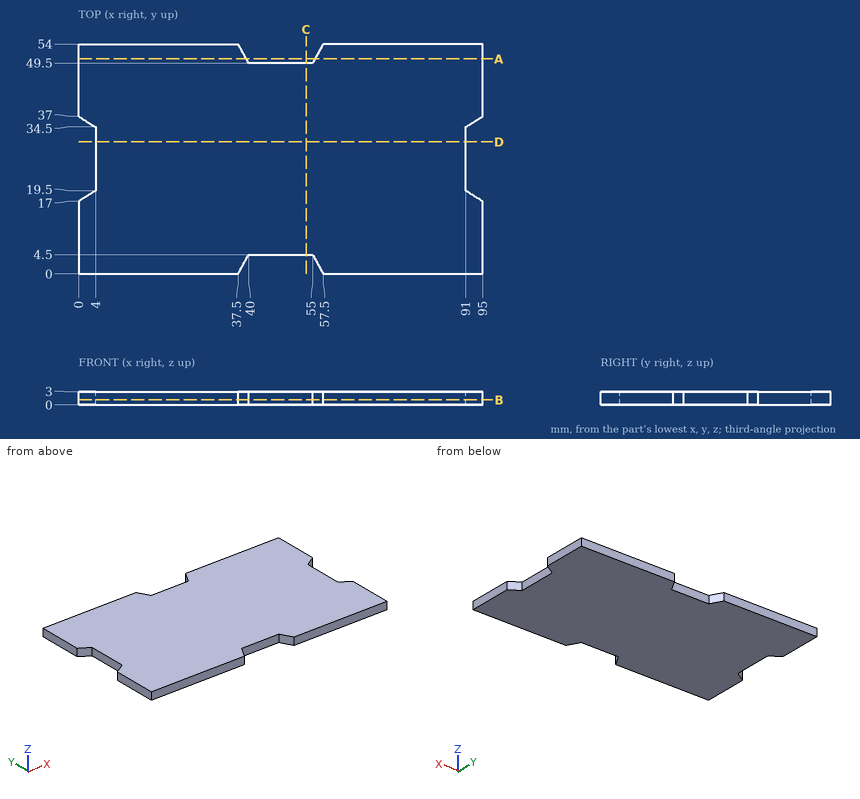
Check sheet for the drawn part. Datum: minimum x, y, z corner. Units: mm. Give positions to 0.01 mm unless a question says otherwise; leave off trailing zeros. Order: outer loops, then holes, each group sorted by start corner. A loop starts at its lowest first (then second) coordinate and runs counter-clockwise, first axis right, second up. Notation, with made-up numbers: (-4.5, 12.5) - (52.5, 12.5) arc R31 cw to (52.5, 48.5) - close; hole circle Ø7 at (52, 10). An arc over 180 degrees is marked (long way). Write item = value, one per line. Start each with the question number.
1) Section check B-B (z = 1.1). Enter the section's corners in (x, y), then the cut area to 3 significant figures.
2) Section check D-D (y = 31). Enter the section's corners in (x, z).
3) Gauge pin test, flat ends, axial feed: pin 1 Ø1.5 at (y, z) = (24.5, 1.5) entering from +X; pin 2 Ø1.5 at (x, z) = (48.5, 1) entering from -Y. Record the tip position at first contact, or that the pin passes through.
4) Scan lines: L1, parallel to Y at x = 50, z = 0.9; L2, parallel to X at y = 33, z = 0.8; L3, parallel to X at y = 3, z = 0.5. Record each from-to range of solid material in increasing order.
5) Section check C-C (x = 53.5). Enter the section's corners in (y, z), then the cut area to 3 significant figures.
6) Section check A-A (y = 50.5). Enter the section's corners in (x, z).
Geometry check:
q1.outline = (0, 0) - (37.5, 0) - (40, 4.5) - (55, 4.5) - (57.5, 0) - (95, 0) - (95, 17) - (91, 19.5) - (91, 34.5) - (95, 37) - (95, 54) - (57.5, 54) - (55, 49.5) - (40, 49.5) - (37.5, 54) - (0, 54) - (0, 37) - (4, 34.5) - (4, 19.5) - (0, 17) - close
q1.area = 4,830 mm2
q2.outline = (4, 0) - (91, 0) - (91, 3) - (4, 3) - close
q3.pin_1 = 91
q3.pin_2 = 4.5
q4.L1 = 4.5 to 49.5
q4.L2 = 4 to 91
q4.L3 = 0 to 39.17, 55.83 to 95
q5.outline = (4.5, 0) - (49.5, 0) - (49.5, 3) - (4.5, 3) - close
q5.area = 135 mm2
q6.outline = (0, 0) - (39.44, 0) - (39.44, 3) - (0, 3) - close; (55.56, 0) - (95, 0) - (95, 3) - (55.56, 3) - close
